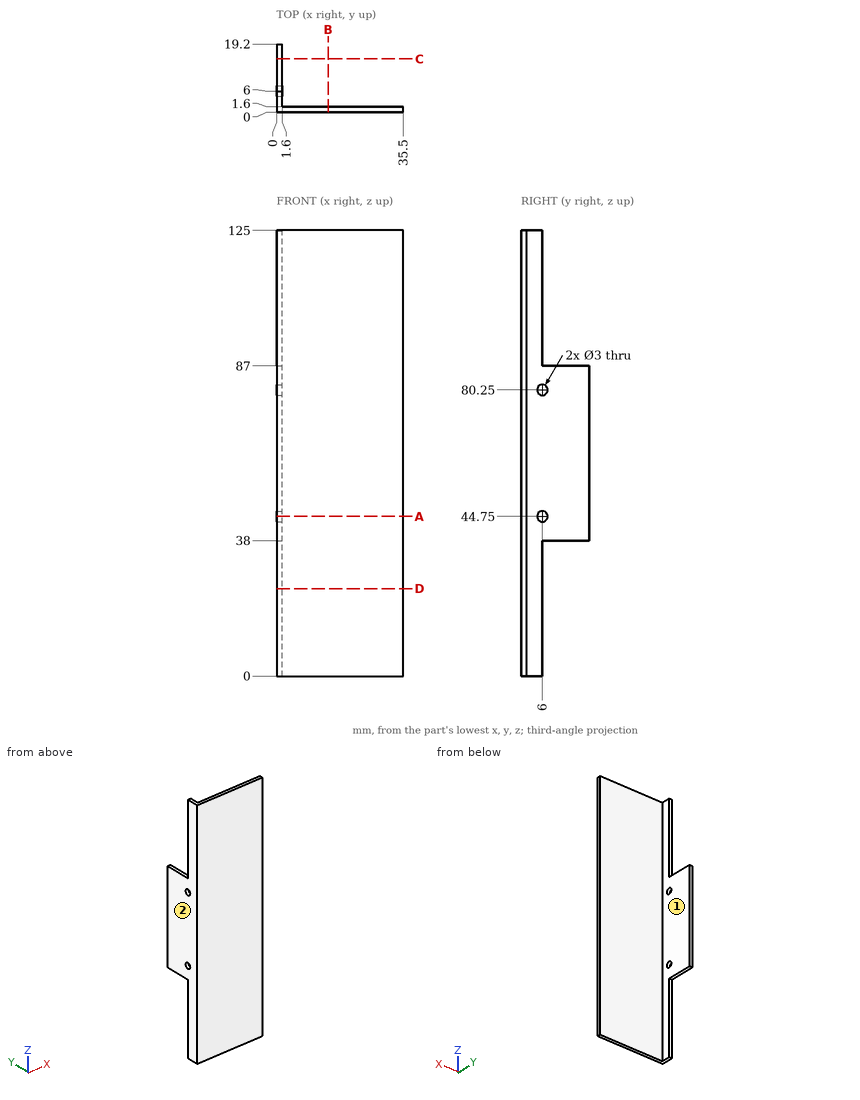
Job drawing, mm, ordinate dimensions from the low corner. One solid piece. A direction names the side the tool comes from. Coordinates: 2 decimals unless noted, no trailing zeros. Write each loop counter-clockwise with the first axis right and the second up, starting at its lowest first coordinate (ties: lowest second). Pieces come first, ordered by that corner, then holes. Notation, with made-up numbers: (0.5, 69.5) - (22.5, 69.5) arc R16 ccw to (22.5, 73.5) - close; hole circle Ø7 at (33.5, 11). An arc over 180 degrees is marked (long way). Use a Markdown table: item, result. Add a question column.
Item 1: Drill centre lines: L1, parallel to Y at x = 1, z = 44.75; L2, parallel to X at y = 4.25, z = 66. Where is each one in solid material? Low to high. Write a range as from..to.
Item 2: Band-saw the part on C-C, the plane y = 15. Give the cut face in (x, z).
Item 3: Flat gauge pins, fed straight in: pin 1 (0.8 mm diameter, centred on x = 1, z = 12, fed in from +Y); pin 2 (5 mm diameter, centred on y = 6, z = 44.75, fed in from +X); pin 3 (1.3 mm diameter, centred on x = 1, y = 14, fed in from +Z); pin 4 (2.5 mm diameter, centred on y = 6, z = 80.25, fed in from +X). Where does each tip first touch, or does it go through?
Item 4: Band-saw the part on B-B, the plane x = 14.5. Give the cut face in (y, z).
Item 5: Band-saw the part on A-A, the plane z = 44.75. Give the cut face in (x, y).
Item 6: Band-saw the part on D-D, the plane z = 24.5. Give the cut face in (x, y).
Item 7: 3-axis set-ups, long thin cutter, end or side, ignore diameter. For the marked faces 1 and 2: which of +Z, -Z, +X, -X, +Y, -Y reach the whole face in a straight line?
Numbers:
| question | item | result |
|---|---|---|
| 1 | L1 | 0..4.5, 7.5..19.2 |
| 1 | L2 | 0..1.6 |
| 2 | outline | (0, 38) - (1.6, 38) - (1.6, 87) - (0, 87) - close |
| 3 | pin 1 | y = 6 |
| 3 | pin 2 | x = 1.6 |
| 3 | pin 3 | z = 87 |
| 3 | pin 4 | through |
| 4 | outline | (0, 0) - (1.6, 0) - (1.6, 125) - (0, 125) - close |
| 5 | outline | (0, 0) - (35.5, 0) - (35.5, 1.6) - (1.6, 1.6) - (1.6, 4.5) - (0, 4.5) - close; (0, 7.5) - (1.6, 7.5) - (1.6, 19.2) - (0, 19.2) - close |
| 6 | outline | (0, 0) - (35.5, 0) - (35.5, 1.6) - (1.6, 1.6) - (1.6, 6) - (0, 6) - close |
| 7 | face 1 | +Z, -Z, +X, +Y |
| 7 | face 2 | +Z, -Z, -X, +Y, -Y |
